Part print with two shaded views. Sizes in mm from the minimum x, y, z corner. Give positions to 0.01 mm unless a question says otherwise; leave off trailing zeros. Loops run counter-clockwise (first coordinate to the right, second up) from the corner with the lowest first, then second, coordinate; pieces in that order, holes last. Notation, with made-up numbers: M 7.5,27.5 L 49.5,27.5 A13 ccw 49.5,35.5 Z; hole C 23,47.25 d10. An arc over 180 degrees is marked long. Answer as a JSON object with one key per item and string values. Group by question number.
1. Slice it at C-C (z = 8.5). List the corners of the cut face in (x, y).
2. Slice it at A-A (x = 9.5). List the corners of the cut face in (y, z) (1 decimal).
3. Slice it at D-D (x = 16.5). List the corners of the cut face in (y, z).
4. Slice it at B-B (y = 0.7). List the corners of the cut face in (x, z) (1 decimal).
5. Drill centre lines: line 1 along X through (y, z) = (0.9, 4) (1 decimal); line 2 along X through (y, z) = (0.5, 3) (1 decimal); line 3 along Z through (x, y) = (10.5, 0.55) (1 decimal). Where is each one in solid material? Low to high. Write a range as [from, to].
6. Drop a flat-ended pin along its axis: pin 1 Ø3 at (x, z) = (53.81, 4.64) entering from -Y. Give the stop position or say it passes through.
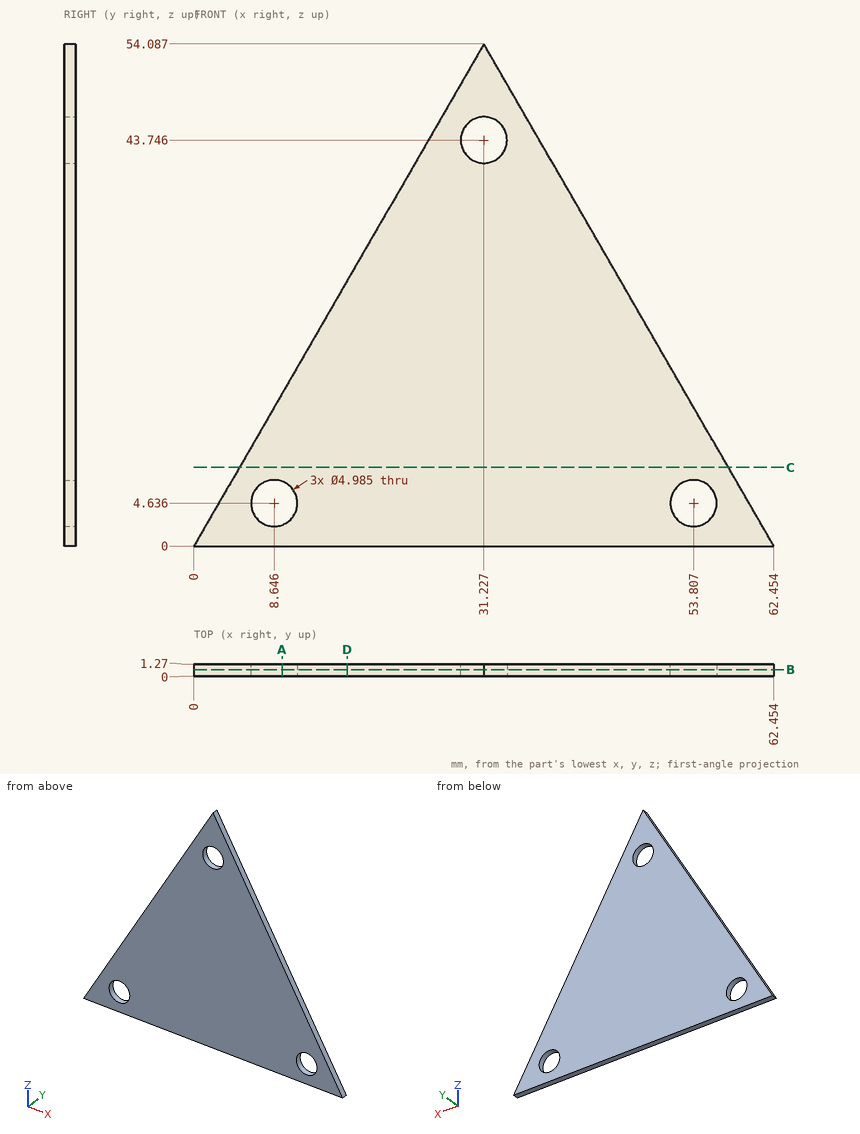
Established:
{
 "1": {"outline": "M 4.91,0 L 57.55,0 L 57.55,1.27 L 4.91,1.27 Z"},
 "2": {"outline": "M 0,0 L 1.3,0 L 1.3,2.3 L 0,2.3 Z; M 0,7 L 1.3,7 L 1.3,16.5 L 0,16.5 Z"},
 "3": {"outline": "M 0,0 L 1.27,0 L 1.27,28.58 L 0,28.58 Z"},
 "4": {"outline": "M 0,0 L 62.5,0 L 31.2,54.1 Z; hole C 8.6,4.6 d5; hole C 31.2,43.7 d5; hole C 53.8,4.6 d5"},
 "5": {"line 1": "x = [2.3, 6.2], [11.1, 51.4], [56.2, 60.1]", "line 2": "x = [1.7, 6.8], [10.5, 51.9], [55.7, 60.7]", "line 3": "z = [0, 3], [6.3, 18.2]"},
 "6": {"pin 1": "passes through"}
}
